Read the model definition and answer for the solid it produces. Units are mm, in the model's axes. Face numbers are marked on the shaded views. A direction names the side the tool comes from. Round coordinates to 2 decimals unless told otherwise and drop trailing zeros. Write each loop counter-clockwise with the first axis right and the second up, starting at its lowest first coordinate (ties: lowest second). Pieces come first, ordered by that corner, then holes. Notation, with made-up numbers: (48, 38.5) -> (91, 38.5) arc R14 ccw to (91, 60.5) -> close; hole circle Ø4 at (2.5, 25). An arc over 180 degrees is marked (long way). Return JSON: item names as keys, results as strings. Group by question number.
(1) For the marked faces 3, 4 and 5, determine the directions among +Z, -Z, +X, -X, +Y, -Y from which every point of the face is accessible in a straight line to the end or side of a thin tool.
(2) A cutting plane is placed at A-A on x = 85. Give the vertices of the cut face in (y, z).
(3) A cutting plane is placed at C-C on z = 10.25. Give the vertices of the cut face in (x, y).
(4) A cutting plane is placed at B-B on x = 0. Give the vertices of the cut face in (y, z).
(5) Straight lines are drawn through the part: line 1 (X direction, y = 5, z = 20.9); line 2 (Y direction, x = 0, z = 14.5); line 3 (X direction, y = 5, z = 8.25). For each, find the intervals that lie inside material, in ascending order.
(6) A cutting plane is placed at D-D on y = -1.5. Give the vertices of the cut face in (x, z).
(7) The mould has two halves that part along X. Classify the marked faces 1 and 2: released by +X, released by -X, zero draft, split by the parting line, or undercut.
(8) Given pin 1 (2 mm diameter, centred on y = 4, z = 10.5, fed in from -X); pin 2 (0.7 mm diameter, centred on y = 2, z = 19.5, fed in from -X); pin 3 (3 mm diameter, centred on x = 0, y = 5, fed in from +Z); pin 4 (1 mm diameter, centred on y = 1, z = 7, fed in from -X), each flat-ended and moving along its own axis, determine where each tip first touches the part or whether it passes through.
Autodesk Fusion 360 part; units mm, degrees
sketch "スケッチ1" plane through (0, 0, 0) normal (0, 0, 1) x (1, 0, 0)
  line L0 (0, 0) -> (85, 0)
  line L1 (85, 0) -> (85, 10)
  line L2 (85, 10) -> (0, 10)
  line L3 (0, 10) -> (0, 0)
  circle A0 centre (85, 5) radius 7.5
  circle A1 centre (0, 5) radius 7.5
  dimension "d1" = 10
  dimension "d2" = 15
  dimension "d3" = 15
extrude "押し出し1" add sketch "スケッチ1" along normal blind 24
sketch "スケッチ2" plane through (0, 0, 24) normal (0, 0, 1) x (-1, 0, 0)
  line L0 (-79.4098, -10) -> (-5.5902, -10)
  arc A0 (-5.5902, -10) -> (-5.5902, 0) centre (0, -5) ccw
  line L1 (-5.5902, 0) -> (-79.4098, 0)
  arc A1 (-79.4098, 0) -> (-79.4098, -10) centre (-85, -5) ccw
  circle A2 centre (-85, -5) radius 3.75
  dimension "d6" = 7.5
extrude "押し出し2" cut sketch "スケッチ2" against normal blind 4.1 contours A2
sketch "スケッチ3" plane through (0, 0, 19.9) normal (0, 0, 1) x (-1, 0, 0)
  circle A0 centre (-85, -5) radius 3.75
  circle A1 centre (-85, -5) radius 3.3
  dimension "d9" = 6.6
extrude "押し出し3" cut sketch "スケッチ3" against normal blind 1.9 contours A1
sketch "スケッチ4" plane through (0, 0, 0) normal (0, 0, -1) x (1, 0, 0)
  line L0 (5.5902, -10) -> (79.4098, -10)
  arc A0 (79.4098, -10) -> (79.4098, 0) centre (85, -5) ccw
  line L1 (79.4098, 0) -> (5.5902, 0)
  arc A1 (5.5902, 0) -> (5.5902, -10) centre (0, -5) ccw
  circle A2 centre (85, -5) radius 2.25
  dimension "d12" = 4.5
extrude "押し出し4" cut sketch "スケッチ4" against normal blind 5.8 contours A2
sketch "スケッチ5" plane through (0, 0, 5.8) normal (0, 0, -1) x (1, 0, 0)
  circle A0 centre (85, -5) radius 2.25
  circle A1 centre (85, -5) radius 1.7
  dimension "d15" = 3.4
extrude "押し出し5" cut sketch "スケッチ5" against normal blind 13 contours A1
sketch "スケッチ6" plane through (0, 0, 0) normal (0, 0, 1) x (1, 0, 0)
  circle A0 centre (0, 5) radius 5
  dimension "d18" = 10
extrude "押し出し6" cut sketch "スケッチ6" along normal blind 4.1
sketch "スケッチ7" plane through (0, 0, 4.1) normal (0, 0, -1) x (1, 0, 0)
  circle A0 centre (0, -5) radius 5
  circle A1 centre (0, -5) radius 6
  dimension "d21" = 12
extrude "押し出し7" cut sketch "スケッチ7" along normal blind 0.85 contours A0 | A1
sketch "スケッチ8" plane through (0, 0, 24) normal (0, 0, 1) x (-1, 0, 0)
  circle A0 centre (-85, -5) radius 3.75
  line L0 (-79.4098, -10) -> (-5.5902, -10)
  arc A1 (-5.5902, -10) -> (-5.5902, 0) centre (0, -5) ccw
  line L1 (-5.5902, 0) -> (-79.4098, 0)
  arc A2 (-79.4098, 0) -> (-79.4098, -10) centre (-85, -5) ccw
  circle A3 centre (0, -5) radius 5
  dimension "d24" = 10
extrude "押し出し8" cut sketch "スケッチ8" against normal blind 4.1 contours A3
sketch "スケッチ9" plane through (0, 0, 19.9) normal (0, 0, 1) x (-1, 0, 0)
  circle A0 centre (0, -5) radius 5
  circle A1 centre (0, -5) radius 6
  dimension "d27" = 12
extrude "押し出し9" cut sketch "スケッチ9" against normal blind 0.85 contours A0 | A1
sketch "スケッチ10" plane through (0, 0, 19.05) normal (0, 0, 1) x (-1, 0, 0)
  circle A0 centre (0, -5) radius 6
  line L0 (-6, -5) -> (6, -5)
  line L1 (6, -5) -> (6, -10)
  line L2 (6, -10) -> (-6, -10)
  line L3 (-6, -10) -> (-6, -5)
sketch "スケッチ11" plane through (0, 0, 0) normal (0, 1, 0) x (1, 0, 0)
  line L0 (6, -19.05) -> (-6.0119, -19.05)
  line L1 (-6.0119, -19.05) -> (-6.0119, -19.9)
  line L2 (-6.0119, -19.9) -> (6, -19.9)
  line L3 (6, -19.9) -> (6, -19.05)
  dimension "d30" = 0.85
extrude "押し出し10" cut sketch "スケッチ11" against normal blind 2.5
sketch "スケッチ12" plane through (0, 0, 0) normal (0, -1, 0) x (1, 0, 0)
  line L0 (-3.3166, 19.05) -> (-3.3166, 19.9)
  line L1 (-3.3166, 19.9) -> (-5.5902, 19.9)
  line L2 (-5.5902, 19.9) -> (-5.5902, 19.05)
  line L3 (-5.5902, 19.05) -> (-3.3166, 19.05)
sketch "スケッチ13" plane through (0, 0, 0) normal (0, -1, 0) x (1, 0, 0)
  line L0 (5.5902, 19.05) -> (5.5902, 0)
  line L1 (5.5902, 0) -> (79.4098, 0)
  line L2 (79.4098, 0) -> (79.4098, 24)
  line L3 (79.4098, 24) -> (5.5902, 24)
  line L4 (5.5902, 24) -> (5.5902, 19.9)
  line L5 (5.5902, 19.9) -> (3.3166, 19.9)
  line L6 (3.3166, 19.9) -> (3.3166, 19.05)
  line L7 (3.3166, 19.05) -> (5.5902, 19.05)
  line L8 (6, 19.05) -> (3.3166, 19.05)
  line L9 (3.3166, 19.05) -> (3.3166, 19.9)
  line L10 (3.3166, 19.9) -> (6, 19.9)
  line L11 (6, 19.9) -> (6, 19.05)
sketch "スケッチ14" plane through (0, 0, 0) normal (0, -1, 0) x (1, 0, 0)
  line L0 (-6, 19.05) -> (-3.3174, 19.05)
  line L1 (-3.3174, 19.05) -> (-3.3174, 19.8997)
  line L2 (-3.3174, 19.8997) -> (-6, 19.8997)
  line L3 (-6, 19.8997) -> (-6, 19.05)
extrude "押し出し11" cut sketch "スケッチ13" sketch "スケッチ14" against normal blind 5 contours L5 L6 L7 L8 L9 L10 L11 of sketch 2
sketch "スケッチ15" plane through (0, 0, 4.1) normal (0, 0, -1) x (1, 0, 0)
  circle A0 centre (0, -5) radius 6
  line L0 (-6, -5) -> (6, -5)
  line L1 (6, -5) -> (6, -10)
  line L2 (6, -10) -> (-6, -10)
  line L3 (-6, -10) -> (-6, -5)
sketch "スケッチ16" plane through (0, 0, 0) normal (0, 1, 0) x (1, 0, 0)
  line L0 (-6, -4.1) -> (6.0025, -4.1)
  line L1 (6.0025, -4.1) -> (6.0025, -3.25)
  line L2 (6.0025, -3.25) -> (-6, -3.25)
  line L3 (-6, -3.25) -> (-6, -4.1)
  dimension "d35" = 0.85
extrude "押し出し12" cut sketch "スケッチ16" against normal blind 2.5
sketch "スケッチ17" plane through (0, 0, 0) normal (0, -1, 0) x (1, 0, 0)
  line L0 (5.5902, 3.25) -> (5.5902, 0)
  line L1 (5.5902, 0) -> (79.4098, 0)
  line L2 (79.4098, 0) -> (79.4098, 24)
  line L3 (79.4098, 24) -> (5.5902, 24)
  line L4 (5.5902, 24) -> (5.5902, 19.9)
  line L5 (5.5902, 19.9) -> (6, 19.9)
  line L6 (6, 19.9) -> (6, 19.05)
  line L7 (6, 19.05) -> (5.5902, 19.05)
  line L8 (5.5902, 19.05) -> (5.5902, 4.1)
  line L9 (5.5902, 4.1) -> (3.3166, 4.1)
  line L10 (3.3166, 4.1) -> (3.3166, 3.25)
  line L11 (3.3166, 3.25) -> (5.5902, 3.25)
  line L12 (6, 4.1) -> (3.3166, 4.1)
  line L13 (3.3166, 4.1) -> (3.3166, 3.25)
  line L14 (3.3166, 3.25) -> (6, 3.25)
  line L15 (6, 3.25) -> (6, 4.1)
  line L16 (-6, 4.1) -> (-3.3175, 4.1)
  line L17 (-3.3175, 4.1) -> (-3.3175, 3.25)
  line L18 (-3.3175, 3.25) -> (-6, 3.25)
  line L19 (-6, 3.25) -> (-6, 4.1)
extrude "押し出し13" cut sketch "スケッチ17" against normal blind 5 contours L9 L10 L11 L12 L13 L14 L15 | L16 L17 L18 L19
sketch "スケッチ18" plane through (0, 0, 4.1) normal (0, 0, -1) x (1, 0, 0)
  circle A0 centre (0, -5) radius 1.7
  dimension "d40" = 3.4
extrude "押し出し14" cut sketch "スケッチ18" against normal blind 15
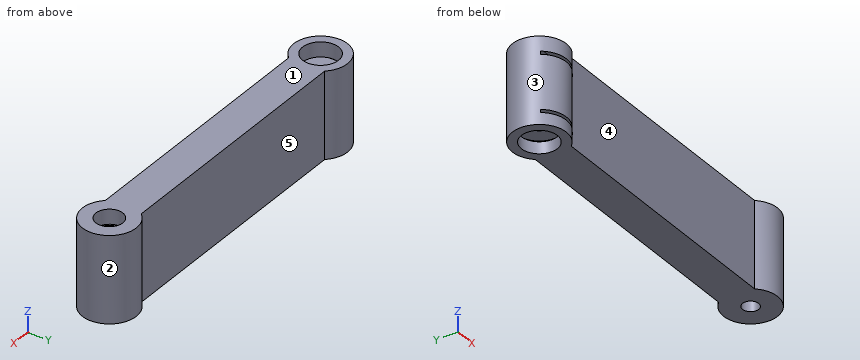
Checks:
{
 "1": {"face 3": "+Z, -Z", "face 4": "+Z, -Z, -Y", "face 5": "+Z, -Z, +Y"},
 "2": {"outline": "(-2.5, 0) -> (2.75, 0) -> (2.75, 5.8) -> (3.3, 5.8) -> (3.3, 18) -> (1.7, 18) -> (1.7, 19.9) -> (1.25, 19.9) -> (1.25, 24) -> (-2.5, 24) -> close; (6.7, 5.8) -> (7.25, 5.8) -> (7.25, 0) -> (12.5, 0) -> (12.5, 24) -> (8.75, 24) -> (8.75, 19.9) -> (8.3, 19.9) -> (8.3, 18) -> (6.7, 18) -> close"},
 "3": {"outline": "(5.59, 0) -> (79.41, 0) arc R7.5 ccw (long way) to (79.41, 10) -> (5.59, 10) arc R7.5 ccw (long way) to start; hole circle Ø3.4 at (0, 5); hole circle Ø3.4 at (85, 5)"},
 "4": {"outline": "(-2.5, 0) -> (0, 0) -> (0, 3.25) -> (-2.5, 3.25) -> close; (-2.5, 4.1) -> (3.3, 4.1) -> (3.3, 19.05) -> (-2.5, 19.05) -> close; (-2.5, 19.9) -> (0, 19.9) -> (0, 24) -> (-2.5, 24) -> close; (6.7, 4.1) -> (11, 4.1) -> (11, 3.25) -> (10, 3.25) -> (10, 0) -> (12.5, 0) -> (12.5, 24) -> (10, 24) -> (10, 19.9) -> (11, 19.9) -> (11, 19.05) -> (6.7, 19.05) -> close"},
 "5": {"line 1": "x = -7.5 to -5, 5 to 81.25, 88.75 to 92.5", "line 2": "y = -2.5 to 3.3, 6.7 to 12.5", "line 3": "x = -7.5 to -1.7, 1.7 to 83.3, 86.7 to 92.5"},
 "6": {"outline": "(-3.74, 0) -> (3.74, 0) -> (3.74, 3.25) -> (-3.74, 3.25) -> close; (-3.74, 4.1) -> (3.74, 4.1) -> (3.74, 19.05) -> (-3.74, 19.05) -> close; (-3.74, 19.9) -> (3.74, 19.9) -> (3.74, 24) -> (-3.74, 24) -> close; (81.26, 0) -> (88.74, 0) -> (88.74, 24) -> (81.26, 24) -> close"},
 "7": {"face 1": "zero draft", "face 2": "undercut"},
 "8": {"pin 1": "stops at x = -7.5", "pin 2": "stops at x = -7.02", "pin 3": "passes through", "pin 4": "stops at x = -6.63"}
}
